Can you work these out from the model? Positions are in its coordinate system, mm. A direction names the side the tool comes from. Give positions to 0.01 mm unless a question says otherwise; leave off trailing zeros. Write each loop counter-clockwise with the first axis right and the second up, starting at its lowest first coordinate (ties: lowest second). Pieces come first, ordered by that corner, then holes. Notation, with made-up numbers: (54, 10.5) -> (105, 10.5) arc R9 cw to (105, 24.5) -> close; hole circle Ø6 at (-27, 6). An arc over 180 degrees is marked (long way). One line per item, written item: value.
from build123d import *
from build123d.topology import SkipClean

# Parameters (mm, degrees)
SKETCH5_R                   = 7.5
CUT_EXTRUDE1_DEPTH          = 90
SKETCH6_R                   = 3.5
CUT_EXTRUDE2_DEPTH          = 20
CIRPATTERN1_COUNT           = 6
SKETCH11_R                  = 3.18
CUT_EXTRUDE4_DEPTH          = 101.105860558
SKETCH23_R                  = 30.48
CUT_EXTRUDE6_DEPTH          = 80.122584091
F_1_4_CLEARANCE_HOLE1_D     = 6.5278
F_1_4_CLEARANCE_HOLE1_DEPTH = 15.4203
F_1_4_CLEARANCE_HOLE1_TIP   = 1.961148974
CHAMFER1_SIZE               = 3.175
SKETCH26_OUTSIDE_W          = 84.718
SKETCH26_OUTSIDE_H          = 84.718
SKETCH26_OUTSIDE_R          = 15
FOR_TURNING_EASE_DEPTH      = 74.878689756
DELETEFACE2_START           = -60.0000001
DELETEFACE2_OUTLINE_R       = 15
DELETEFACE2_OUTLINE_R_2     = 10.16
DELETEFACE2_DEPTH           = 60.0000001
CHAMFER3_SIZE               = 1.6
SKETCH30_R                  = 21.082
SKETCH30_R_2                = 19.05
GASKET_GROOVE_DEPTH         = 1.27
MOVE_START                  = 6.35
MOVE_FACE3_OUTLINE_R        = 30.48
MOVE_FACE3_OUTLINE_R_2      = 3.2639
MOVE_FACE3_DEPTH            = 7.62


with BuildPart() as part:
    # Sketch1 → Revolve1 (revolve)
    with BuildSketch(Plane(origin=(0, 0, 0), x_dir=(0, 0, -1), z_dir=(1, 0, 0))):
        Polygon((0, 30.35), (12.7, 30.35), (12.7, 6.35), (30.48, 6.35), (30.48, 0), (15.68, 0), (10.16, -20.600920458), (10.16, -60), (0, -60), align=None)
    revolve(axis=Axis((0, 0, 0), (0, 1, 0)))

    # Sketch5 → Cut-Extrude1 (cut)
    with BuildSketch(Plane.XZ.offset(60)):
        with Locations(Location((0, 0, 0), (0, 0, 270))):
            Circle(SKETCH5_R)
    extrude(amount=-CUT_EXTRUDE1_DEPTH, mode=Mode.SUBTRACT)

    # Sketch6 → Cut-Extrude2 (cut, symmetric)
    with BuildSketch(Plane.XY):
        with Locations((0, 16.659966967)):
            Circle(SKETCH6_R)
    cut_extrude2 = extrude(amount=CUT_EXTRUDE2_DEPTH, both=True, mode=Mode.SUBTRACT)

    # CirPattern1: Cut-Extrude2 ×6 about axis
    cirpattern1_axis = Axis((0, 30.35, 0), (0, -1, 0))
    for i in range(1, CIRPATTERN1_COUNT):
        add(cut_extrude2.rotate(cirpattern1_axis, i * 360 / CIRPATTERN1_COUNT), mode=Mode.SUBTRACT)

    # Sketch11 → Cut-Extrude4 (cut, through all)
    with BuildSketch(Plane(origin=(0, 30.35, 0), x_dir=(1, 0, 0), z_dir=(0, 1, 0))):
        with Locations(Location((0, 0, 0), (0, 0, 270))):
            Circle(SKETCH11_R)
    extrude(amount=-CUT_EXTRUDE4_DEPTH, mode=Mode.SUBTRACT)

    # Sketch23 → Cut-Extrude6 (cut, through all)
    with BuildSketch(Plane(origin=(0, 6.35, 0), x_dir=(1, 0, 0), z_dir=(0, 1, 0))):
        with Locations(Location((0, 0, 0), (0, 0, 90))):
            Circle(SKETCH23_R)
    extrude(amount=CUT_EXTRUDE6_DEPTH, mode=Mode.SUBTRACT)

    # 1/4 Clearance Hole1
    with Locations(Plane(origin=(0, 6.35, 0), x_dir=(1, 0, 0), z_dir=(0, 1, 0))):
        with Locations((-20.151174843, 15.462540297), (23.466540126, 9.720159182), (20.151174843, -15.462540297), (-23.466540126, -9.720159182)):
            Hole(F_1_4_CLEARANCE_HOLE1_D / 2, depth=F_1_4_CLEARANCE_HOLE1_DEPTH)
            with Locations((0, 0, -(F_1_4_CLEARANCE_HOLE1_DEPTH + F_1_4_CLEARANCE_HOLE1_TIP / 2))):  # 118° drill point
                Cone(0, F_1_4_CLEARANCE_HOLE1_D / 2, F_1_4_CLEARANCE_HOLE1_TIP, mode=Mode.SUBTRACT)

    # Chamfer1
    chamfer1_edges = [part.edges().sort_by_distance(p)[0] for p in [
        (0, 6.35, 7.5),
    ]]
    chamfer(chamfer1_edges, length=CHAMFER1_SIZE)

    # Sketch26 outside → for-turning-ease (cut, through all)
    with BuildSketch(Plane.XZ):
        Rectangle(SKETCH26_OUTSIDE_W, SKETCH26_OUTSIDE_H)
        with Locations(Location((0, 0, 0), (0, 0, 90))):
            Circle(SKETCH26_OUTSIDE_R, mode=Mode.SUBTRACT)
    extrude(amount=FOR_TURNING_EASE_DEPTH, mode=Mode.SUBTRACT)

    # DeleteFace2: read off the stored shape, not the designer's step
    # DeleteFace2 outline → DeleteFace2 (cut)
    with BuildSketch(Plane(origin=(0, 0, 0), x_dir=(1, 0, 0), z_dir=(0, 1, 0)).offset(DELETEFACE2_START)):
        Circle(DELETEFACE2_OUTLINE_R)
        Circle(DELETEFACE2_OUTLINE_R_2, mode=Mode.SUBTRACT)
    extrude(amount=DELETEFACE2_DEPTH, mode=Mode.SUBTRACT)

    # Chamfer3
    # the kernel refuses this chamfer: 1.6 mm, written as the material it adds along each edge
    with BuildSketch(Plane(origin=(0, 0, 0), x_dir=(1, 0, 0), z_dir=(0, 0, 1))) as chamfer3_piece_1:
        Polygon((10.16 + CHAMFER3_SIZE, 0), (10.16, -CHAMFER3_SIZE), (10.16, 0), align=None)
    revolve(axis=Axis((0, 0, 0), (0, 1, 0)))

    # Sketch30 → gasket_groove (cut)
    with BuildSketch(Plane.XZ):
        with Locations(Location((0, 0, 0), (0, 0, 270))):
            Circle(SKETCH30_R)
        with Locations(Location((0, 0, 0), (0, 0, 270))):
            Circle(SKETCH30_R_2, mode=Mode.SUBTRACT)
    extrude(amount=-GASKET_GROOVE_DEPTH, mode=Mode.SUBTRACT)

    # Move Face3: read off the stored shape, not the designer's step
    # Move Face3 outline → Move Face3 (add)
    with SkipClean():  # the faces are left unmerged after this step: merging them gives an invalid solid
        with BuildSketch(Plane(origin=(0, 0, 0), x_dir=(1, 0, 0), z_dir=(0, 1, 0)).offset(MOVE_START)):
            Circle(MOVE_FACE3_OUTLINE_R)
            with Locations((-23.466540126, -9.720159182)):
                Circle(MOVE_FACE3_OUTLINE_R_2, mode=Mode.SUBTRACT)
            with Locations((20.151174843, -15.462540297)):
                Circle(MOVE_FACE3_OUTLINE_R_2, mode=Mode.SUBTRACT)
            with Locations((-20.151174843, 15.462540297)):
                Circle(MOVE_FACE3_OUTLINE_R_2, mode=Mode.SUBTRACT)
            with Locations((23.466540126, 9.720159182)):
                Circle(MOVE_FACE3_OUTLINE_R_2, mode=Mode.SUBTRACT)
        extrude(amount=MOVE_FACE3_DEPTH)
    add(part.part.scale(1), mode=Mode.REPLACE)  # the faces are merged on a copy

    # Move Face3 2 outline → Move Face3 2 (revolve, cut)
    with SkipClean():  # the faces are left unmerged after this step: merging them gives an invalid solid
        with BuildSketch(Plane.XY):
            Polygon((18.295, 13.97), (0, 13.97), (0, 6.35), (10.675, 6.35), align=None)
        revolve(axis=Axis((0, 0, 0), (0, 1, 0)), mode=Mode.SUBTRACT)


solid = part.part
1) Will these pins go through, and if not, where does the flat tip stop? pin 1 (1.5 mm diameter, centred on x = 6.5, y = -22, fed in from +Z); pin 2 (17 mm diameter, centred on x = 0, z = 0, fed in from -Y); pin 3 (6 mm diameter, centred on x = 23.47, z = -9.72, fed in from +Y); pin 4 (8.5 mm diameter, centred on x = 20.15, z = 15.46, fed in from -Y).
Answer list:
pin 1: stops at z = 8.38
pin 2: stops at y = -60
pin 3: passes through
pin 4: stops at y = 0
2) If we section it at B-B (y = 9.5): Write out the boundary of the cut face in (x, z) (3 decimals), and give its area (3 significant figures).
Answer list:
outline: circle Ø60.96 at (0, 0); hole circle Ø6.528 at (-23.467, 9.72); hole circle Ø6.528 at (-20.151, -15.463); hole circle Ø27.65 at (0, 0); hole circle Ø6.528 at (20.151, 15.463); hole circle Ø6.528 at (23.467, -9.72)
area: 2,180 mm^2
3) If we section it at C-C (z = 26.5): Write out the boundary of the cut face in (x, y).
Answer list:
outline: (-15.06, 0) -> (15.06, 0) -> (15.06, 13.97) -> (-15.06, 13.97) -> close
4) We'd pull the mould along Z, two halves only. Please class faces 1 (the face through (-5.36, -31.21, -8.63)), 2 (the face through (6, -60, 5)), 3 (the face through (-11, 1.27, 16)): released by +Z, released by -Z, zero draft, split by the parting line, or undercut.
Answer list:
face 1: split by the parting line
face 2: zero draft
face 3: undercut
5) If we section it at A-A (y = -10.5): Write out the boundary of the cut face in (x, z), and give its area (3 significant figures).
Answer list:
outline: circle Ø20.32 at (0, 0); hole circle Ø15 at (0, 0)
area: 148 mm^2
6) For faces 4 (the face through (13.1, 13.97, 13.1)), 5 (the face through (-21, 0, -6)), which set-ups out of +Z, -Z, +X, -X, +Y, -Y let a thin tool reach every point of the face, with its end or its side?
Answer list:
face 4: +Z, -Z, +X, -X, +Y
face 5: -Y
7) I need wall thicknesses on L1, parallel to Z at x = 0.5, y = -11; L2, parallel to Z at x = 8.5, y = 0.5; L3, parallel to X at y = 0.5, z = 1. Which ranges of each line are inside material? Lowest first, please.
Answer list:
L1: z = -10.15 to -7.48, 7.48 to 10.15
L2: z = -29.27 to -19.29, -17.05 to 17.05, 19.29 to 29.27
L3: x = -30.46 to -21.06, -19.02 to -7.43, 7.43 to 19.02, 21.06 to 30.46
